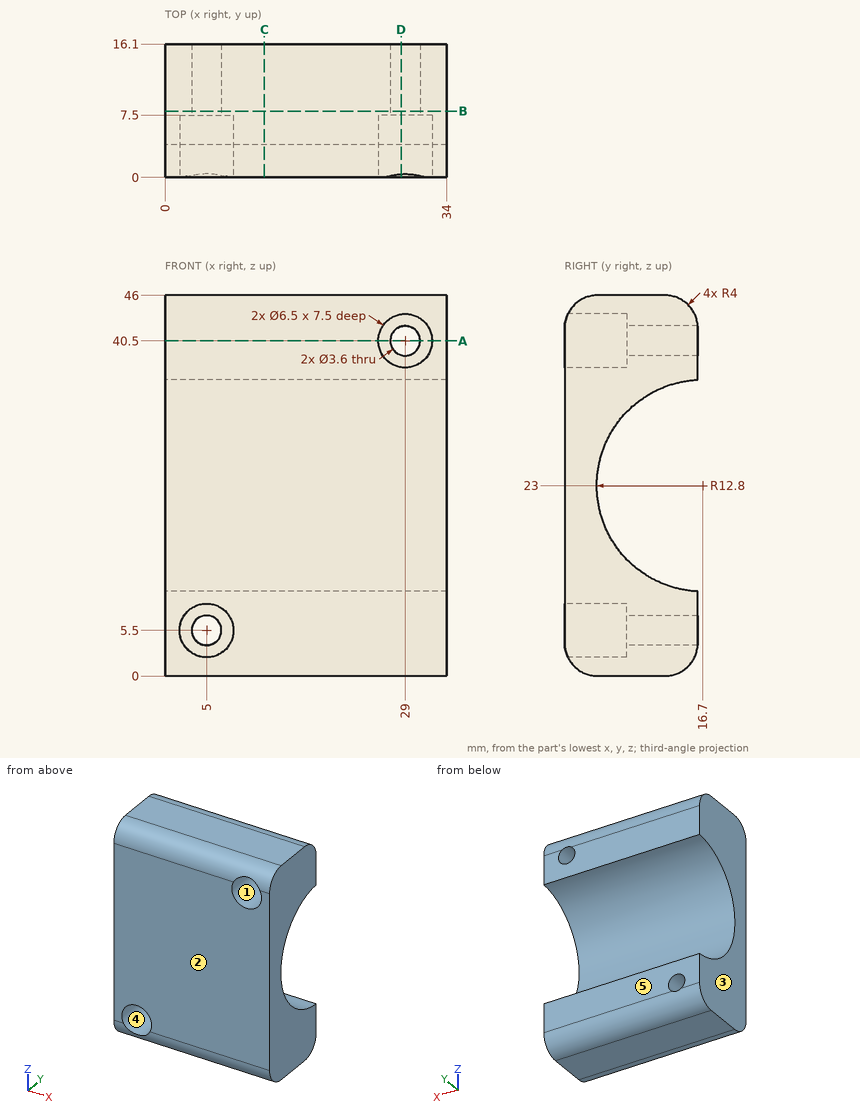
Study the drawing (mm; zero at the part's minimum x, y, z) and answer. A direction names the side the tool comes from. Give positions to 0.01 mm unless a question says otherwise; leave off trailing zeros. Loops run counter-clockwise (first coordinate to the right, second up) from the corner with the lowest first, then second, coordinate; pieces in that order, holes last. Notation, with made-up numbers: (-33.75, -29) -> (20.25, -29) arc R20 ccw to (20.25, -10) -> close; hole circle Ø4 at (39, 7). An arc over 180 degrees is marked (long way). Use a Markdown table: item, result. Add a question column.
1) The part is cut by section D-D, the plane x = 28.5. Determine the outline of the cut face in (y, z), plus the area to 3 significant figures.
2) For a pull along X with two mould halves and no side action, classify the marked faces 1, 2 and 3 as +X half, -X half, draft (parallel to the pull), parting line (faces both ways), or undercut.
3) The part is cut by section C-C, the plane x = 12. Determine the outline of the cut face in (y, z), plus the area to 3 significant figures.
4) The part is cut by section A-A, the plane z = 40.5. Determine the outline of the cut face in (x, y), plus the area to 3 significant figures.
5) Each of these flat-tipped pins is pushed along its axis until it touches: P1, Ø3, axis at x = 5, z = 5.5, coming from the +Y side; P2, Ø5, axis at x = 5.5, z = 5.5, coming from the -Y side; P3, Ø1.5, axis at x = 10, z = 18, coming from the +Y side. Where does it stop, or does it pass through?
6) The part is cut by section B-B, the plane y = 8. Determine the outline of the cut face in (x, z).
7) Consider line 1 along X through (y, z) = (2.5, 5.5); line 2 along X through (y, z) = (10, 40.5); line 3 along Z through (x, y) = (29, 14). Determine where each line is inside the solid, lowest interval first.
8) Which of the six approach directions +Z, -Z, +X, -X, +Y, -Y give full straight-line access (tool end or side, diameter ignored) to the marked faces 4 and 5?
Reported:
| question | item | result |
|---|---|---|
| 1 | outline | (0, 4) arc R4 ccw to (4, 0) -> (12.1, 0) arc R4 ccw to (16.1, 4) -> (16.1, 10.21) arc R12.8 cw to (16.1, 35.79) -> (16.1, 38.77) -> (7.5, 38.77) -> (7.5, 37.29) -> (0, 37.29) -> close; (0.38, 43.71) -> (7.5, 43.71) -> (7.5, 42.23) -> (16.09, 42.23) arc R4 ccw to (12.1, 46) -> (4, 46) arc R4 ccw to start |
| 1 | area | 407 mm^2 |
| 2 | face 1 | undercut |
| 2 | face 2 | draft |
| 2 | face 3 | -X half |
| 3 | outline | (0, 4) arc R4 ccw to (4, 0) -> (12.1, 0) arc R4 ccw to (16.1, 4) -> (16.1, 10.21) arc R12.8 cw to (16.1, 35.79) -> (16.1, 42) arc R4 ccw to (12.1, 46) -> (4, 46) arc R4 ccw to (0, 42) -> close |
| 3 | area | 485 mm^2 |
| 4 | outline | (0, 0) -> (25.75, 0) -> (25.75, 7.5) -> (27.2, 7.5) -> (27.2, 16.1) -> (0, 16.1) -> close; (30.8, 7.5) -> (32.25, 7.5) -> (32.25, 0) -> (34, 0) -> (34, 16.1) -> (30.8, 16.1) -> close |
| 4 | area | 468 mm^2 |
| 5 | P1 | passes through |
| 5 | P2 | stops at y = 7.5 |
| 5 | P3 | stops at y = 5.26 |
| 6 | outline | (0, 0) -> (34, 0) -> (34, 13.61) -> (0, 13.61) -> close; (0, 32.39) -> (34, 32.39) -> (34, 46) -> (0, 46) -> close; hole circle Ø3.6 at (5, 5.5); hole circle Ø3.6 at (29, 40.5) |
| 7 | line 1 | x = 0 to 1.75, 8.25 to 34 |
| 7 | line 2 | x = 0 to 27.2, 30.8 to 34 |
| 7 | line 3 | z = 0.48 to 10.49, 35.51 to 38.7, 42.3 to 45.52 |
| 8 | face 4 | -Y |
| 8 | face 5 | +Z, -Z, +X, -X, +Y |
